Build history of the part. All positions in model axes, mm. A direction names the side the tool comes from. Coordinates: 2 decimals unless noted, no trailing zeros. Write each loop counter-clockwise with the first axis right and the second up, starting at its lowest first coordinate (ties: lowest second). Pieces come first, ordered by that corner, then holes. Notation, with made-up numbers: (46.5, -9) -> (100.5, -9) arc R7 cw to (100.5, 1) -> close; hole circle Ø3 at (-32, 2.5). An arc over 180 degrees is marked (long way). Write each question's results on one line, items separated by ' | '. Start each with the question number.
Q1. Saw through at C-C on x = 350. Give the cut face in (y, z).
Q2. Saw through at B-B on z = 4. Give the cut face in (x, y).
Q3. Saw through at D-D on y = 121. Give the cut face in (x, z).
Q4. Drop flat-ended pins along their axis: pin 1 Ø6 at (x, z) = (554, 2.5) entering from -Y; pin 2 Ø25 at (y, z) = (464, 10) entering from +X; pin 3 Ø10 at (x, z) = (761, 13.5) entering from -Y. Give the stop position or say it passes through.
Q5. Two-plate mould, pull along X, no slides. Class faces 4 (the face through (944.297, 6.014, 0.35)), 5 (the face through (750, 50, 0)), 6 (the face through (99, 500, 0)): released by +X, released by -X, zero draft, split by the parting line, or undercut.
Q6. Saw through at A-A on x = 100. Give the cut face in (y, z), and give its area (3 significant figures).
Q7. Tool access for faces 1 (the face through (138.153, 112.015, -0.35)), 2 (the face through (303, 400, 0)), 3 (the face through (744.297, 93.986, 0.35)): list every direction of +Z, -Z, +X, -X, +Y, -Y with a clear straight run to the whole face (end or side of a thin tool).
Q8. Drill centre lines: line 1 (Y direction, x = 100, z = -6); line 2 (X direction, y = 47.5, z = -12.5); line 3 (Y direction, x = 79, z = 15.5). Where is each one in solid material? Low to high.
from build123d import *

# Parameters (mm, degrees)
SKETCH1_R           = 30
SKETCH1_R_2         = 40
SKETCH1_R_3         = 25
BOSS_EXTRUDE1_DEPTH = 25


with BuildPart() as part:
    # Sketch1 → Boss-Extrude1 (new body, symmetric)
    with BuildSketch(Plane.XY):
        with BuildLine():
            Line((200, 480), (200, 420))
            ThreePointArc((200, 420), (205.857864376, 405.857864376), (220, 400))
            Line((220, 400), (388.241879306, 400))
            ThreePointArc((388.241879306, 400), (398.249452654, 397.316133393), (405.571126809, 389.984847569))
            ThreePointArc((405.571126809, 389.984847569), (551.290675458, 246.959096298), (750, 200))
            Line((750, 200), (930, 200))
            ThreePointArc((930, 200), (944.142135624, 194.142135624), (950, 180))
            Line((950, 180), (950, 20))
            ThreePointArc((950, 20), (944.142135624, 5.857864376), (930, 0))
            Line((930, 0), (770, 0))
            ThreePointArc((770, 0), (755.857864376, 5.857864376), (750, 20))
            Line((750, 20), (750, 80))
            ThreePointArc((750, 80), (744.142135624, 94.142135624), (730, 100))
            Line((730, 100), (220, 100))
            ThreePointArc((220, 100), (205.857864376, 94.142135624), (200, 80))
            Line((200, 80), (200, 20))
            ThreePointArc((200, 20), (194.142135624, 5.857864376), (180, 0))
            Line((180, 0), (20, 0))
            ThreePointArc((20, 0), (5.857864376, 5.857864376), (0, 20))
            Line((0, 20), (0, 480))
            ThreePointArc((0, 480), (5.857864376, 494.142135624), (20, 500))
            Line((20, 500), (180, 500))
            ThreePointArc((180, 500), (194.142135624, 494.142135624), (200, 480))
        make_face()
        with Locations((100, 400)):
            Circle(SKETCH1_R, mode=Mode.SUBTRACT)
        with Locations((100, 100)):
            Circle(SKETCH1_R_2, mode=Mode.SUBTRACT)
        with Locations((350, 250)):
            Circle(SKETCH1_R_3, mode=Mode.SUBTRACT)
        with Locations((850, 100)):
            Circle(SKETCH1_R_2, mode=Mode.SUBTRACT)
    extrude(amount=BOSS_EXTRUDE1_DEPTH, both=True)


solid = part.part
Returned:
1) outline: (100, -25) -> (225, -25) -> (225, 25) -> (100, 25) -> close; (275, -25) -> (400, -25) -> (400, 25) -> (275, 25) -> close
2) outline: (0, 20) arc R20 ccw to (20, 0) -> (180, 0) arc R20 ccw to (200, 20) -> (200, 80) arc R20 cw to (220, 100) -> (730, 100) arc R20 cw to (750, 80) -> (750, 20) arc R20 ccw to (770, 0) -> (930, 0) arc R20 ccw to (950, 20) -> (950, 180) arc R20 ccw to (930, 200) -> (750, 200) arc R380 cw to (405.57, 389.98) arc R20 ccw to (388.24, 400) -> (220, 400) arc R20 cw to (200, 420) -> (200, 480) arc R20 ccw to (180, 500) -> (20, 500) arc R20 ccw to (0, 480) -> close; hole circle Ø80 at (100, 100); hole circle Ø60 at (100, 400); hole circle Ø50 at (350, 250); hole circle Ø80 at (850, 100)
3) outline: (0, -25) -> (65.96, -25) -> (65.96, 25) -> (0, 25) -> close; (134.04, -25) -> (815.96, -25) -> (815.96, 25) -> (134.04, 25) -> close; (884.04, -25) -> (950, -25) -> (950, 25) -> (884.04, 25) -> close
4) pin 1: stops at y = 100 | pin 2: stops at x = 200 | pin 3: stops at y = 0.4
5) face 4: released by +X | face 5: undercut | face 6: zero draft
6) outline: (0, -25) -> (60, -25) -> (60, 25) -> (0, 25) -> close; (140, -25) -> (370, -25) -> (370, 25) -> (140, 25) -> close; (430, -25) -> (500, -25) -> (500, 25) -> (430, 25) -> close | area: 18,000 mm2
7) face 1: +Z, -Z | face 2: +Z, -Z, +X, +Y | face 3: +Z, -Z, -Y
8) line 1: y = 0 to 60, 140 to 370, 430 to 500 | line 2: x = 0 to 200, 750 to 950 | line 3: y = 0 to 65.96, 134.04 to 378.58, 421.42 to 500
